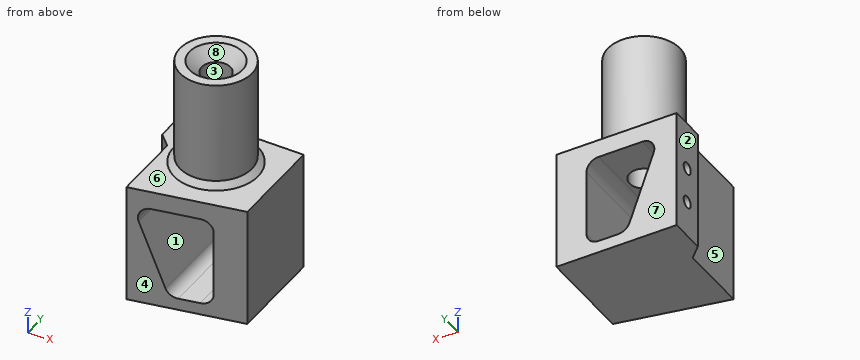
```python
from build123d import *

# Parameters (mm, degrees)
SKETCH1_R                                       = 3
BOSS_EXTRUDE1_DEPTH                             = 10
SKETCH1_3_R                                     = 3
BOSS_EXTRUDE2_DEPTH                             = 9
CUT_EXTRUDE1_DEPTH                              = 10
SKETCH2_R                                       = 0.5
CUT_EXTRUDE2_DEPTH                              = 5
CHAMFER1_SIZE                                   = 0.5
CSK_FOR_M2_FLAT_HEAD_MACHINE_SCREW1_D           = 2.4
CSK_FOR_M2_FLAT_HEAD_MACHINE_SCREW1_DEPTH       = 10.5
CSK_FOR_M2_FLAT_HEAD_MACHINE_SCREW1_CSINK_D     = 4.4
CSK_FOR_M2_FLAT_HEAD_MACHINE_SCREW1_CSINK_ANGLE = 90


with BuildPart() as part:
    # Sketch1 → Boss-Extrude1 (new body)
    # profile 1 of 3: a face of its own
    with BuildSketch(Plane.XY):
        Polygon((-4, 1), (-4, -4.8), (5, -3), (5, 5), (-4, 5), align=None)
        with Locations((0, 1.099019514)):
            Circle(SKETCH1_R, mode=Mode.SUBTRACT)
    # profile 2 of 3: a face of its own
    with BuildSketch(Plane.XY):
        Polygon((-5, 2), (-4, 1), (-4, 5), (-5, 5), align=None)
    # profile 3 of 3: a face of its own
    with BuildSketch(Plane.XY):
        with Locations((0, 1.099019514)):
            Circle(SKETCH1_R)
    extrude(amount=-BOSS_EXTRUDE1_DEPTH)

    # Sketch1<3> → Boss-Extrude2 (add)
    with BuildSketch(Plane.XY):
        with Locations((0, 1.099019514)):
            Circle(SKETCH1_3_R)
    extrude(amount=BOSS_EXTRUDE2_DEPTH)

    # Sketch5 → Cut-Extrude1 (cut)
    with BuildSketch(Plane(origin=(0, 5, 0), x_dir=(1, 0, 0), z_dir=(0, 1, 0))):
        with BuildLine():
            Line((1.5, 9), (-0.140385722, 9))
            ThreePointArc((-0.140385722, 9), (-0.713962158, 8.819152044), (-1.080078342, 8.342020143))
            Line((-1.080078342, 8.342020143), (-3.081914631, 2.842020143))
            ThreePointArc((-3.081914631, 2.842020143), (-2.961374054, 1.926423564), (-2.14222201, 1.5))
            Line((-2.14222201, 1.5), (0, 1.5))
            Line((0, 1.5), (1.5, 1.5))
            ThreePointArc((1.5, 1.5), (2.207106781, 1.792893219), (2.5, 2.5))
            Line((2.5, 2.5), (2.5, 4))
            Line((2.5, 4), (2.5, 8))
            ThreePointArc((2.5, 8), (2.207106781, 8.707106781), (1.5, 9))
        make_face()
    extrude(amount=-CUT_EXTRUDE1_DEPTH, mode=Mode.SUBTRACT)

    # Sketch2 → Cut-Extrude2 (cut)
    with BuildSketch(Plane.ZY.offset(5)):
        with Locations(Location((-7, 3.5, 0), (0, 0, 270))):
            Circle(SKETCH2_R)
        with Locations(Location((-4, 3.5, 0), (0, 0, 270))):
            Circle(SKETCH2_R)
    extrude(amount=-CUT_EXTRUDE2_DEPTH, mode=Mode.SUBTRACT)

    # Chamfer1
    chamfer1_edges = [part.edges().sort_by_distance(p)[0] for p in [
        (-3, 1.099019514, 0),
    ]]
    chamfer(chamfer1_edges, length=CHAMFER1_SIZE)

    # CSK for M2 Flat Head Machine Screw1
    with Locations(Plane.XY.offset(9)):
        with Locations((0, 1.099019514)):
            CounterSinkHole(CSK_FOR_M2_FLAT_HEAD_MACHINE_SCREW1_D / 2, CSK_FOR_M2_FLAT_HEAD_MACHINE_SCREW1_CSINK_D / 2, depth=CSK_FOR_M2_FLAT_HEAD_MACHINE_SCREW1_DEPTH, counter_sink_angle=CSK_FOR_M2_FLAT_HEAD_MACHINE_SCREW1_CSINK_ANGLE)


solid = part.part
```
Source: CAD feature listing. Evaluate the final solid. Frame: model axes, mm. Face numbers are marked on the shaded views. A direction names the side the tool comes from. Round coordinates to 2 decimals unless told otherwise and drop trailing zeros. Order: outer loops, then holes, each group sorted by start corner. A loop starts at its lowest first (then second) coordinate and runs counter-clockwise, first axis right, second up. Notation, with made-up numbers: (45, 81) -> (82, 81) arc R11 ccw to (82, 94) -> close; hole circle Ø11 at (86.25, -26.5). An arc over 180 degrees is marked (long way). Use CSV: the item, a comma, the result in double quotes.
(1) Section D-D on z = 5.5. Return the cut outline in (x, y), and give its area (3 significant figures).
Report:
outline,"circle Ø6 at (0, 1.1); hole circle Ø2.4 at (0, 1.1)"
area,"23.8 mm^2"
(2) Ray query, L1, parallel to Z at x = -3.8, y = 3.5; L2, parallel to Y at x = 0, z = -1.25; L3, parallel to X at y = -2.75, z = -7.5. Return the intervals inside material, ascending.
Report:
L1,"-10 to -7.5, -6.5 to -4.5, -3.5 to 0"
L2,"-4 to -0.1, 2.3 to 5"
L3,"-4 to -1.39, 2.5 to 5"
(3) Access query for the marked faces 1, 2, 3, 4 and 5. Directions: +Z, -Z, +X, -X, +Y, -Y. A direction counts if a zero-diameter tool reaches every point of the face in a straight line with its end or side. Return the directions, or none.
Report:
face 1,"+Y, -Y"
face 2,"+Z, -Z, -X, +Y, -Y"
face 3,"+Z"
face 4,"+Z, -Z, +X, -Y"
face 5,"+Z, -Z, -X, -Y"
(4) Section A-A on z = -7. Return the cut outline in (x, y), and give its area (3 significant figures).
Report:
outline,"(-5, 2) -> (-4, 1) -> (-4, -4.8) -> (-1.57, -4.31) -> (-1.57, 3) -> (-5, 3) -> close; (-5, 4) -> (-1.57, 4) -> (-1.57, 5) -> (-5, 5) -> close; (2.5, -3.5) -> (5, -3) -> (5, 5) -> (2.5, 5) -> close"
area,"43.9 mm^2"
(5) Section B-B on x = 4.25. Return the cut outline in (y, z).
Report:
outline,"(-3.15, -10) -> (5, -10) -> (5, 0) -> (-3.15, 0) -> close"
(6) First-contact query: pin 1 Ø1.5 at (x, z) = (-1.5, 1) entering from -Y; pin 2 Ø1.6 at (y, z) = (-0.5, -4) entering from -X; pin 3 Ø5 at (y, z) = (-3, 5.5) entering from +X. Flat tips, straight axial feed; report the tip coordinate or a pass-through.
Report:
pin 1,"y = -1.85"
pin 2,"x = -4"
pin 3,"x = 2.54"
(7) Section C-C on z = -4. Return the cut outline in (x, y).
Report:
outline,"(-5, 2) -> (-4, 1) -> (-4, -4.8) -> (-2.66, -4.53) -> (-2.66, 3) -> (-5, 3) -> close; (-5, 4) -> (-2.66, 4) -> (-2.66, 5) -> (-5, 5) -> close; (2.5, -3.5) -> (5, -3) -> (5, 5) -> (2.5, 5) -> close"
(8) Pull-direction query (Y, two-part tool) for the marked faces 6, 7 and 8; classes: +Y half, -Y half, draft (parallel to the pull), parting line (faces both ways), or undercut.
Report:
face 6,"draft"
face 7,"+Y half"
face 8,"undercut"
